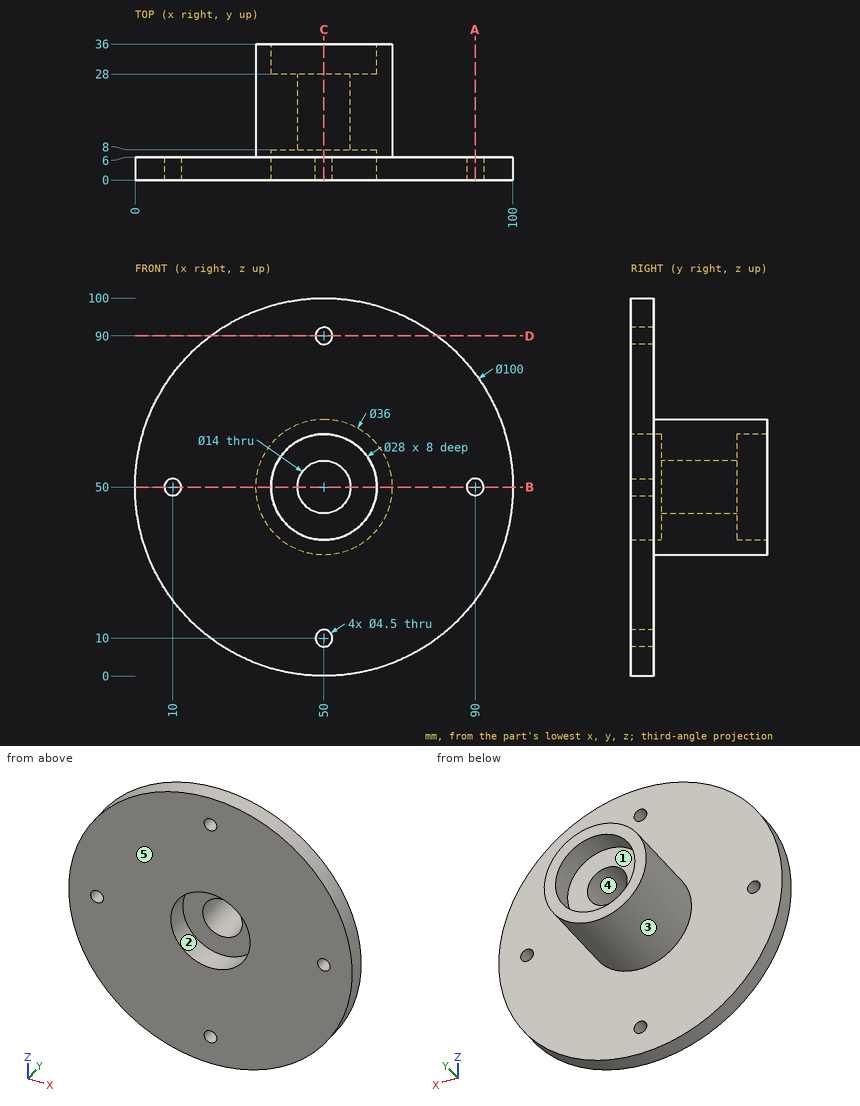
Check sheet for the drawn part. Datum: minimum x, y, z corner. Units: mm. A direction names the side the tool comes from. Coordinates: 2 decimals unless noted, no trailing zeros. Order: outer loops, then holes, each group sorted by start corner. A loop starts at its lowest first (then second) coordinate and runs counter-clockwise, first axis right, second up. Notation, with made-up numbers: (-7.5, 41.5) -> (-1.5, 41.5) arc R26 cw to (-1.5, 80.5) -> close; hole circle Ø5 at (86.5, 18). An arc over 180 degrees is marked (long way). Use a Markdown table: item, result. Add a question column.
1. Cross-section at A-A (x = 90). Enter the section's corners in (y, z).
2. Cross-section at C-C (x = 50). Enter the section's corners in (y, z), and give its area (3 significant figures).
3. Mould release check, pull along X, two halves, no side actions. Record for the marked faces 3, 4 and 5: pulls with the +X half, pulls with the -X half, needs draft (parallel to the pull), parting line crosses it, or undercut.
4. Cross-section at B-B (z = 50). Enter the section's corners in (x, y), and give its area (3 significant figures).
5. Go/stop test with flat-tipped pins: pin 1 Ø7 at (x, z) = (50, 10) entering from +Y; pin 2 Ø1 at (y, z) = (32.5, 47.5) entering from +X; pin 3 Ø12 at (x, y) = (56.5, 24) entering from -Z. Record where each tip stops, or that it passes through.
6. Material ranges on L1, parallel to X at y = 2.5, z = 50; L2, parallel to Z at x = 50.5, y = 10.5; L3, parallel to X at y = 33.25, z = 50, recorded low to high.
7. Set-up check for the marked faces 1 and 2: record each of +Z, -Z, +X, -X, +Y, -Y from which the full face is reachable in a straight line by a thin tool's end or side.
8. Cross-section at D-D (z = 90). Enter the section's corners in (x, y), and give its area (3 significant figures).
Filled sheet:
| question | item | result |
|---|---|---|
| 1 | outline | (0, 20) -> (6, 20) -> (6, 47.75) -> (0, 47.75) -> close; (0, 52.25) -> (6, 52.25) -> (6, 80) -> (0, 80) -> close |
| 2 | outline | (0, 0) -> (6, 0) -> (6, 7.75) -> (0, 7.75) -> close; (0, 12.25) -> (6, 12.25) -> (6, 32) -> (36, 32) -> (36, 36) -> (28, 36) -> (28, 43) -> (8, 43) -> (8, 36) -> (0, 36) -> close; (0, 64) -> (8, 64) -> (8, 57) -> (28, 57) -> (28, 64) -> (36, 64) -> (36, 68) -> (6, 68) -> (6, 87.75) -> (0, 87.75) -> close; (0, 92.25) -> (6, 92.25) -> (6, 100) -> (0, 100) -> close |
| 2 | area | 898 mm2 |
| 3 | face 3 | parting line crosses it |
| 3 | face 4 | undercut |
| 3 | face 5 | needs draft |
| 4 | outline | (0, 0) -> (7.75, 0) -> (7.75, 6) -> (0, 6) -> close; (12.25, 0) -> (36, 0) -> (36, 8) -> (43, 8) -> (43, 28) -> (36, 28) -> (36, 36) -> (32, 36) -> (32, 6) -> (12.25, 6) -> close; (57, 8) -> (64, 8) -> (64, 0) -> (87.75, 0) -> (87.75, 6) -> (68, 6) -> (68, 36) -> (64, 36) -> (64, 28) -> (57, 28) -> close; (92.25, 0) -> (100, 0) -> (100, 6) -> (92.25, 6) -> close |
| 4 | area | 898 mm2 |
| 5 | pin 1 | y = 6 |
| 5 | pin 2 | x = 67.89 |
| 5 | pin 3 | z = 32.01 |
| 6 | L1 | 0 to 7.75, 12.25 to 36, 64 to 87.75, 92.25 to 100 |
| 6 | L2 | 32.01 to 43.02, 56.98 to 67.99 |
| 6 | L3 | 32 to 36, 64 to 68 |
| 7 | face 1 | +Y |
| 7 | face 2 | -Y |
| 8 | outline | (20, 0) -> (47.75, 0) -> (47.75, 6) -> (20, 6) -> close; (52.25, 0) -> (80, 0) -> (80, 6) -> (52.25, 6) -> close |
| 8 | area | 333 mm2 |
